Could you check a few things on this drawing? It's one solid part, dimensions in mm from its lowest x, y, z. Give positions to 0.01 mm unless a question says otherwise; leave off trailing zeros. Order: outer loops, then holes, each group sorted by start corner. A loop starts at its lowest first (then second) coordinate and runs counter-clockwise, first axis right, second up.
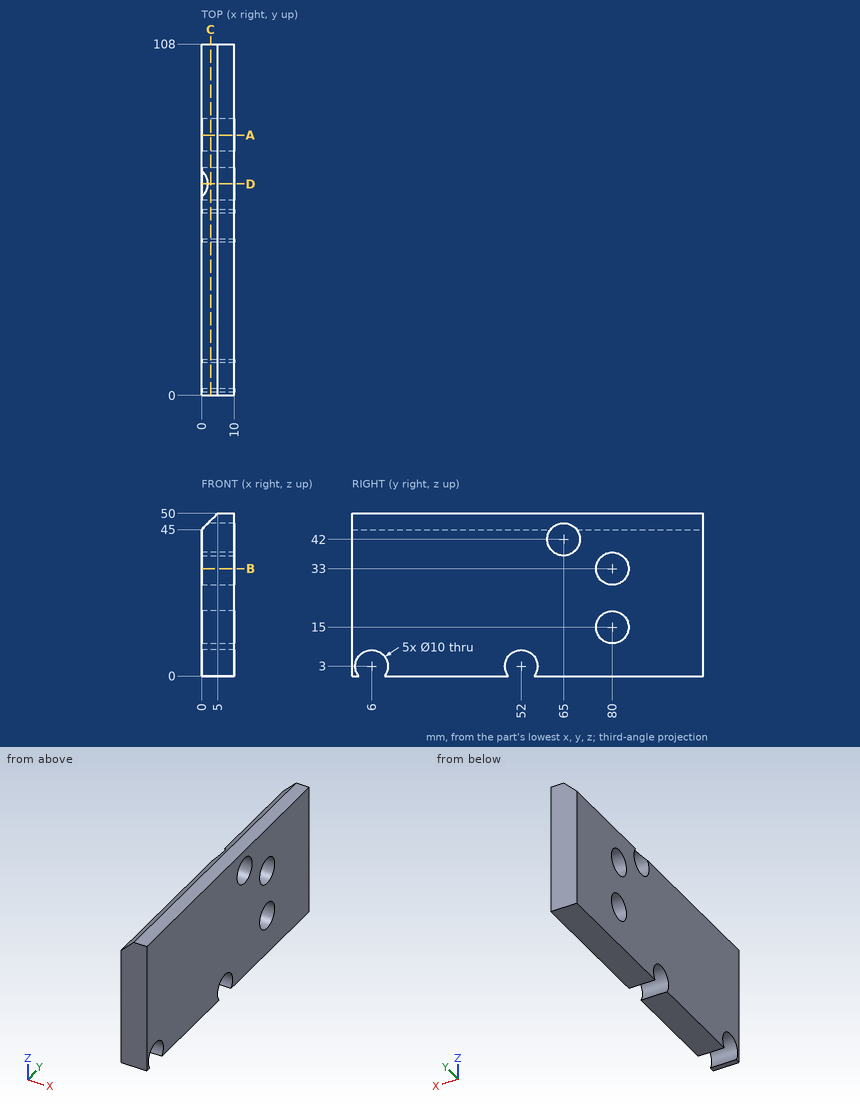
1) Suppose I cut it at D-D (y = 65). Please give me the cut outline in (x, z), and give its area (4 significant figures).
2) Suppose I cut it at A-A (y = 80). Please give me the cut outline in (x, z).
3) Suppose I cut it at B-B (z = 33). Please give me the cut outline in (x, y).
4) Suppose I cut it at C-C (x = 2.75). Please give me the cut outline in (y, z).
5) If I drill on line 1 (Y direction, x = 4.25, z = 6); line 2 (Y direction, x = 5.75, z = 3); line 3 (Z direction, x = 7.75, y = 80), over which ranges is the centre line in solid material (lowest first)?
Results:
1. outline: (0, 0) - (10, 0) - (10, 37) - (0, 37) - close; (2, 47) - (10, 47) - (10, 50) - (5, 50) - close
1. area: 389.5 mm2
2. outline: (0, 0) - (10, 0) - (10, 10) - (0, 10) - close; (0, 20) - (10, 20) - (10, 28) - (0, 28) - close; (0, 38) - (10, 38) - (10, 50) - (5, 50) - (0, 45) - close
3. outline: (0, 0) - (10, 0) - (10, 75) - (0, 75) - close; (0, 85) - (10, 85) - (10, 108) - (0, 108) - close
4. outline: (0, 0) - (2, 0) arc R5 cw (long way) to (10, 0) - (48, 0) arc R5 cw (long way) to (56, 0) - (108, 0) - (108, 47.75) - (0, 47.75) - close; hole circle Ø10 at (65, 42); hole circle Ø10 at (80, 15); hole circle Ø10 at (80, 33)
5. line 1: y = 0 to 2, 10 to 48, 56 to 108
5. line 2: y = 0 to 1, 11 to 47, 57 to 108
5. line 3: z = 0 to 10, 20 to 28, 38 to 50
